Part model, mm, in its own coordinate system. Round coordinates to 2 decimals unless told otherwise and drop trailing zeros. Order: outer loops, then holes, each group sorted by start corner. A loop starts at its lowest first (then second) coordinate and runs counter-clockwise, first axis right, second up. Notation, with made-up numbers: (-18.5, -28) - (32.5, -28) arc R23 cw to (32.5, 10) - close; hole circle Ø8 at (87.25, -13). An arc over 180 degrees is marked (long way). Answer as a JSON object with one key per item and string values.
```python
from build123d import *

# Parameters (mm, degrees)
SKETCH1_W           = 61
SKETCH1_H           = 85
BOSS_EXTRUDE1_DEPTH = 3.5
SKETCH2_R           = 1.5
CUT_EXTRUDE1_DEPTH  = 3.5
SKETCH3_R           = 1.5
CUT_EXTRUDE2_DEPTH  = 3.5
FILLET1_R           = 3


with BuildPart() as part:
    # Sketch1 → Boss-Extrude1 (new body)
    with BuildSketch(Plane(origin=(0, 0, 0), x_dir=(1, 0, 0), z_dir=(0, 1, 0))):
        Rectangle(SKETCH1_W, SKETCH1_H)
    extrude(amount=BOSS_EXTRUDE1_DEPTH)

    # Sketch2 → Cut-Extrude1 (cut)
    with BuildSketch(Plane(origin=(0, 3.5, 0), x_dir=(1, 0, 0), z_dir=(0, 1, 0))):
        with Locations(Location((-27.5, 39.5, 0), (0, 0, 270))):
            Circle(SKETCH2_R)
        with Locations(Location((27.5, 39.5, 0), (0, 0, 270))):
            Circle(SKETCH2_R)
        with Locations(Location((-27.5, -39.5, 0), (0, 0, 270))):
            Circle(SKETCH2_R)
        with Locations(Location((27.5, -39.5, 0), (0, 0, 270))):
            Circle(SKETCH2_R)
    extrude(amount=-CUT_EXTRUDE1_DEPTH, mode=Mode.SUBTRACT)

    # Sketch3 → Cut-Extrude2 (cut)
    with BuildSketch(Plane(origin=(0, 3.5, 0), x_dir=(1, 0, 0), z_dir=(0, 1, 0))):
        with Locations(Location((-13, 17, 0), (0, 0, 270))):
            Circle(SKETCH3_R)
        with Locations(Location((13, -17, 0), (0, 0, 270))):
            Circle(SKETCH3_R)
        with Locations(Location((13, 17, 0), (0, 0, 270))):
            Circle(SKETCH3_R)
        with Locations(Location((-13, -17, 0), (0, 0, 270))):
            Circle(SKETCH3_R)
    extrude(amount=-CUT_EXTRUDE2_DEPTH, mode=Mode.SUBTRACT)

    # Fillet1
    fillet1_edges = [part.edges().sort_by_distance(p)[0] for p in [
        (30.5, 1.75, 42.5),
        (-30.5, 1.75, 42.5),
        (-30.5, 1.75, -42.5),
        (30.5, 1.75, -42.5),
    ]]
    fillet(fillet1_edges, radius=FILLET1_R)


solid = part.part
```
Item 1: Drop flat-ended pins along their axis: P1, Ø3.5, axis at x = 27.5, z = -39.5, coming from the -Y side; P2, Ø2.5, axis at x = -13, z = -17, coming from the -Y side. Give the stop position or say it passes through.
Taken from the geometry:
{"P1": "y = 0", "P2": "through"}
Item 2: Probe L1, parallel to X at y = 0.85, z = 17; L2, parallel to X at y = 1.6, z = -39.5. List the from-to ranges inside material, lowest first. Write a range as from..to.
Taken from the geometry:
{"L1": "-30.5..-14.5, -11.5..11.5, 14.5..30.5", "L2": "-30.5..-29, -26..26, 29..30.5"}
Item 3: Cut at A-A (x = 13). Write the cut outline in (y, z).
Taken from the geometry:
{"outline": "(0, -42.5) - (3.5, -42.5) - (3.5, -18.5) - (0, -18.5) - close; (0, -15.5) - (3.5, -15.5) - (3.5, 15.5) - (0, 15.5) - close; (0, 18.5) - (3.5, 18.5) - (3.5, 42.5) - (0, 42.5) - close"}
Item 4: Cut at B-B (z = 17). Write the cut outline in (x, y).
Taken from the geometry:
{"outline": "(-30.5, 0) - (-14.5, 0) - (-14.5, 3.5) - (-30.5, 3.5) - close; (-11.5, 0) - (11.5, 0) - (11.5, 3.5) - (-11.5, 3.5) - close; (14.5, 0) - (30.5, 0) - (30.5, 3.5) - (14.5, 3.5) - close"}
Item 5: Two-plate mould, pull along Z, no slides. Class faces 1 (the flat face through (0, 0, -1)), 2 (the flat face through (0, 2, -42.5)), 3 (the cylindrical face through (-12.93, 1.77, 15.5)), 4 (the cylindrical face through (29.6, 1.77, 41.64)): pulls with the +Z half, pulls with the -Z half, needs draft (parallel to the pull), parting line crosses it, or undercut.
Taken from the geometry:
{"face 1": "needs draft", "face 2": "pulls with the -Z half", "face 3": "undercut", "face 4": "pulls with the +Z half"}
